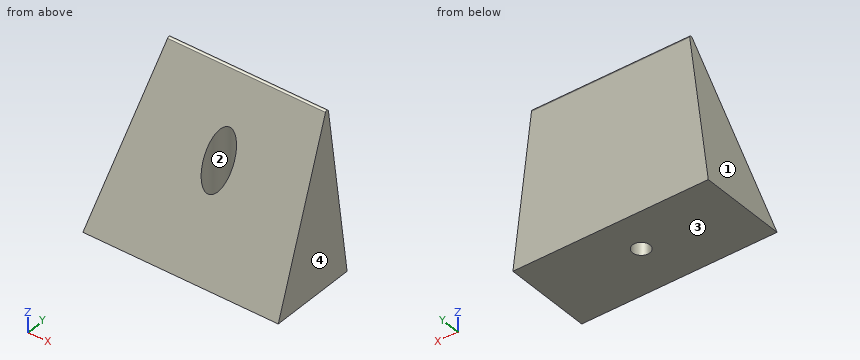
from build123d import *

# Parameters (mm, degrees)
F1_DEPTH       = 45
F3_DEPTH       = 50.001
F3_DEPTH_BACK  = 50.001
F6_D           = 8.8
F6_CBORE_D     = 14.25
F6_CBORE_DEPTH = 8
F5_R           = 7.125
F7_DEPTH       = 80
F8_R           = 1


with BuildPart() as f1:
    # F0 (on Front) → F1 (new body)
    with BuildSketch(Plane.XZ):
        Polygon((-50, 0), (50, 0), (40, 80), (-40, 80), align=None)
    extrude(amount=F1_DEPTH)

    # F2 (on Right) → F3 (cut, two sides)
    with BuildSketch(Plane.YZ) as f3_sk:
        Polygon((-45, 0), (0, 80), (-45, 80), align=None)
    extrude(amount=-F3_DEPTH, mode=Mode.SUBTRACT)
    extrude(f3_sk.sketch, amount=F3_DEPTH_BACK, mode=Mode.SUBTRACT)

    # F6 (through all)
    with Locations(Plane.XY.offset(25)):
        with Locations((0, -20)):
            CounterBoreHole(F6_D / 2, F6_CBORE_D / 2, F6_CBORE_DEPTH)

    # F5 (on offset) → F7 (cut)
    with BuildSketch(Plane.XY.offset(25)):
        with Locations((0, -20)):
            Circle(F5_R)
    extrude(amount=F7_DEPTH, mode=Mode.SUBTRACT)

    # F8
    f8_edges = [f1.edges().sort_by_distance(p)[0] for p in [
        (0, 0, 80),
    ]]
    fillet(f8_edges, radius=F8_R)


solid = f1.part
CAD build for the part. Positions are in the model's coordinates, mm. Face numbers are marked on the shaded views. Give positions to 0.01 mm unless a question says otherwise; leave off trailing zeros. Order: outer loops, then holes, each group sorted by start corner. A loop starts at its lowest first (then second) coordinate and runs counter-clockwise, first axis right, second up. Notation, with made-up numbers: (49, 60.25) -> (92, 60.25) arc R28 cw to (92, 79.25) -> close; hole circle Ø8 at (29.25, 74.5). An arc over 180 degrees is marked (long way). Return JSON: item names as keys, results as strings.
Q1. Saw through at A-A (x = 0). Write the cut outline in (y, z) (1 decimal), then the cut area to 3 significant figures.
Working result:
{"outline": "(-45, 0) -> (-24.4, 0) -> (-24.4, 17) -> (-27.1, 17) -> (-27.1, 31.8) -> close; (-15.6, 0) -> (0, 0) -> (0, 76.2) arc R1 ccw to (-1.9, 76.7) -> (-12.9, 57.1) -> (-12.9, 17) -> (-15.6, 17) -> close", "area": "1,260 mm²"}
Q2. Mould opens along X. For the marked faces 1, 2, 3 and 4 say: pulls with the +X half, pulls with the -X half, needs draft (parallel to the pull), parting line crosses it, or undercut.
Working result:
{"face 1": "pulls with the -X half", "face 2": "undercut", "face 3": "needs draft", "face 4": "pulls with the +X half"}
Q3. Saw through at C-C (z = 10.5). Write the cut outline in (x, y), then the cut area to 3 significant figures.
Working result:
{"outline": "(-48.69, -39.09) -> (48.69, -39.09) -> (48.69, 0) -> (-48.69, 0) -> close; hole circle Ø8.8 at (0, -20)", "area": "3,750 mm²"}
Q4. Saw through at B-B (y = -20). Write the cut outline in (x, z) (3 decimals).
Working result:
{"outline": "(-50, 0) -> (-4.4, 0) -> (-4.4, 17) -> (-7.125, 17) -> (-7.125, 44.444) -> (-44.444, 44.444) -> close; (4.4, 0) -> (50, 0) -> (44.444, 44.444) -> (7.125, 44.444) -> (7.125, 17) -> (4.4, 17) -> close"}
Q5. Flat gauge pins, fed straight in: pin 1 (12 mm diameter, centred on x = 11.5, y = -31.5, fed in from +Z); pin 2 (3 mm diameter, centred on x = 39, y = -26.5, fed in from -Z); pin 3 (11.5 mm diameter, centred on x = 1.5, y = -18.5, fed in from +Z). Where does each tip first touch, or does it go through?
Working result:
{"pin 1": "z = 34.67", "pin 2": "z = 0", "pin 3": "z = 57.33"}
Q6. Drill centre lines: line 1 (Y direction, x = 0, z = 47) (3 decimals); line 2 (X direction, y = -20, z = 33) (3 decimals); line 3 (X direction, y = -15, z = 44). Where is each one in solid material? Low to high.
Working result:
{"line 1": "-12.875 to 0", "line 2": "-45.875 to -7.125, 7.125 to 45.875", "line 3": "-44.5 to -5.08, 5.08 to 44.5"}
